```python
from build123d import *

# Parameters (mm, degrees)
BOSS_EXTRUDE2_DEPTH = 21.59
CUT_EXTRUDE1_DEPTH  = 17.78
BOSS_EXTRUDE4_DEPTH = 2.54
SKETCH8_R           = 1.905
CUT_EXTRUDE2_DEPTH  = 2.54
BOSS_EXTRUDE6_DEPTH = 2.54
FILLET1_R           = 2.54
SKETCH13_W          = 19.05
SKETCH13_H          = 2.54
CUT_EXTRUDE5_DEPTH  = 1.27
CUT_EXTRUDE6_DEPTH  = 1.27
SKETCH16_W          = 19.05
SKETCH16_H          = 2.54
CUT_EXTRUDE7_DEPTH  = 1.27
SKETCH17_R          = 8.89
BOSS_EXTRUDE7_DEPTH = 21.844
FILLET2_R           = 2.54


with BuildPart() as part:
    # Sketch3 → Boss-Extrude2 (new body)
    with BuildSketch(Plane.XY):
        with BuildLine():
            Line((-22.77090231, 76.154735329), (22.77090231, 76.154735329))
            ThreePointArc((22.77090231, 76.154735329), (24.597640016, 75.379566583), (25.309393487, 73.527199387))
            Line((25.309393487, 73.527199387), (22.858491178, 2.452464058))
            ThreePointArc((22.858491178, 2.452464058), (22.084831254, 0.713262294), (20.32, 0))
            Line((20.32, 0), (-20.32, 0))
            ThreePointArc((-20.32, 0), (-22.084831254, 0.713262294), (-22.858491178, 2.452464058))
            Line((-22.858491178, 2.452464058), (-25.309393487, 73.527199387))
            ThreePointArc((-25.309393487, 73.527199387), (-24.597640016, 75.379566583), (-22.77090231, 76.154735329))
        make_face()
    extrude(amount=BOSS_EXTRUDE2_DEPTH)

    # Sketch4 → Cut-Extrude1 (cut)
    with BuildSketch(Plane.XY.offset(21.59)):
        with BuildLine():
            Line((-19.541270744, 73.614735329), (20.141804619, 73.614735329))
            ThreePointArc((20.141804619, 73.614735329), (21.968542325, 72.839566583), (22.680295797, 70.987199387))
            Line((22.680295797, 70.987199387), (20.404569365, 4.992462187))
            ThreePointArc((20.404569365, 4.992462187), (19.630909441, 3.253260423), (17.866078187, 2.539998129))
            Line((17.866078187, 2.539998129), (-18.061159176, 2.539998129))
            ThreePointArc((-18.061159176, 2.539998129), (-19.78310781, 3.39559701), (-20.412160003, 5.212586245))
            Line((-20.412160003, 5.212586245), (-22.687990425, 71.210339105))
            ThreePointArc((-22.687990425, 71.210339105), (-21.690891162, 73.166710129), (-19.541270744, 73.614735329))
        make_face()
    extrude(amount=-CUT_EXTRUDE1_DEPTH, mode=Mode.SUBTRACT)

    # Sketch7 → Boss-Extrude4 (add)
    with BuildSketch(Plane.XY.offset(21.59)):
        Polygon((-21.717608556, 43.069831723), (-8.531459132, 43.069831723), (-8.531459132, 32.909831723), (-21.367256671, 32.909831723), align=None)
        Polygon((8.531459132, 32.909831723), (21.367256671, 32.909831723), (21.717608556, 43.069831723), (8.531459132, 43.069831723), align=None)
    extrude(amount=-BOSS_EXTRUDE4_DEPTH)

    # Sketch8 → Cut-Extrude2 (cut)
    with BuildSketch(Plane.XY.offset(21.59)):
        with Locations((-15.036945873, 37.989831723)):
            Circle(SKETCH8_R)
        with Locations((15.237744036, 37.820383377)):
            Circle(SKETCH8_R)
    extrude(amount=-CUT_EXTRUDE2_DEPTH, mode=Mode.SUBTRACT)

    # Sketch10 → Boss-Extrude6 (add)
    with BuildSketch(Plane.XY.offset(10.795)):
        with BuildLine():
            Line((-19.48633529, 73.614735329), (20.196740073, 73.614735329))
            ThreePointArc((20.196740073, 73.614735329), (22.023477783, 72.839566579), (22.73523125, 70.987199377))
            Line((22.73523125, 70.987199377), (20.459504542, 4.992462177))
            ThreePointArc((20.459504542, 4.992462177), (19.685844615, 3.253260419), (17.921013365, 2.539998129))
            Line((17.921013365, 2.539998129), (-18.006223999, 2.539998129))
            ThreePointArc((-18.006223999, 2.539998129), (-19.816312644, 3.37520138), (-20.468700556, 5.258914571))
            Line((-20.468700556, 5.258914571), (-22.744530979, 71.256667431))
            ThreePointArc((-22.744530979, 71.256667431), (-21.694916693, 73.236386905), (-19.48633529, 73.614735329))
        make_face()
    extrude(amount=BOSS_EXTRUDE6_DEPTH)

    # Fillet1
    fillet1_edges = [part.edges().sort_by_distance(p)[0] for p in [
        (24.083942332, 37.989831723, 0),
        (22.084831254, 0.713262294, 0),
        (0, 0, 0),
        (-22.084831254, 0.713262294, 0),
        (-24.083942332, 37.989831723, 0),
        (-24.597640016, 75.379566583, 0),
        (0, 76.154735329, 0),
        (24.597640016, 75.379566583, 0),
    ]]
    fillet(fillet1_edges, radius=FILLET1_R)

    # Sketch13 → Cut-Extrude5 (cut)
    with BuildSketch(Plane(origin=(22.746873247, -0.784390739, 0), x_dir=(0, 0, -1), z_dir=(0.999405975, -0.034462969, 0))):
        with Locations((-12.065, 47.745550873)):
            Rectangle(SKETCH13_W, SKETCH13_H)
    extrude(amount=-CUT_EXTRUDE5_DEPTH, mode=Mode.SUBTRACT)

    # Sketch14 → Cut-Extrude6 (cut)
    with BuildSketch(Plane(origin=(0, 0, 0), x_dir=(-1, 0, 0), z_dir=(0, 0, -1))):
        Polygon((-21.897084419, 48.274526929), (21.853290434, 48.274526929), (21.853290434, 45.734526929), (-21.809496448, 45.734526929), align=None)
    extrude(amount=-CUT_EXTRUDE6_DEPTH, mode=Mode.SUBTRACT)

    # Sketch16 → Cut-Extrude7 (cut)
    with BuildSketch(Plane(origin=(-22.746873247, -0.784390739, 0), x_dir=(0, 0, 1), z_dir=(-0.999405975, -0.034462969, 0))):
        with Locations((12.065, 47.745550873)):
            Rectangle(SKETCH16_W, SKETCH16_H)
    extrude(amount=-CUT_EXTRUDE7_DEPTH, mode=Mode.SUBTRACT)

    # Sketch17 → Boss-Extrude7 (add)
    with BuildSketch(Plane(origin=(0, 0, 0), x_dir=(-1, 0, 0), z_dir=(0, 0, -1))):
        with Locations((-0.010948496, 60.944631129)):
            Circle(SKETCH17_R)
    extrude(amount=BOSS_EXTRUDE7_DEPTH)

    # Fillet2
    fillet2_edges = [part.edges().sort_by_distance(p)[0] for p in [
        (8.900948496, 60.944631129, 0),
    ]]
    fillet(fillet2_edges, radius=FILLET2_R)


solid = part.part
```
Here's how the part is built. I have some questions about the finished solid (model axes, mm). A direction names the side the tool comes from. Give positions to 0.01 mm unless a question says otherwise; leave off trailing zeros. Order: outer loops, then holes, each group sorted by start corner. A loop starts at its lowest first (then second) coordinate and runs counter-clockwise, first axis right, second up. Notation, with made-up numbers: (58.25, -7.75) -> (103.25, -7.75) arc R28 cw to (103.25, 22.25) -> close; hole circle Ø11 at (3, -27.5). An arc over 180 degrees is marked (long way). Use CSV: the item, a comma, the result in double quotes. Start each with the question number.
Item 1: On a 3-axis mill with a long thin cutter (end or side, diameter ignored), from which of +Z, -Z, +X, -X, +Y, -Y can I reach the whole of each face in a straight line? I mean faces 4 (the flat face through (10, 55, 0)), 5 (the cylindrical face through (-23.338, 38.514, 0.724)), 6 (the cylindrical face through (19.65, 3.27, 17.52)), 7 (the cylindrical face through (19.65, 3.27, 7.35)). Say none if no direction works.
Item 2: I'm going to push flat-ended pins straight in: P1, Ø1.4, axis at x = 4, z = 1, coming from the +Y side; P2, Ø3, axis at x = -15, y = 37, coming from the -Z side; P3, Ø1.3, axis at y = 36, z = 19.5, coming from the +X side. Where does each tip first touch, or does it pass through?
Item 3: Suppose I cut it at A-A (x = 12.5). List the corners of the cut face in (y, z) for me (3 decimals).
Item 4: Suppose I cut it at D-D (z = -14). List the corners of the cut face in (x, y) for me, and give its area (3 significant figures).
Item 5: Suppose I cut it at B-B (z = 5). List the corners of the cut face in (x, y) for me.
Item 6: If I drill on probe 1 along Y at (x, z) = (5, 8); probe 2 along Z at (x, y) = (8, 27) (3 decimals); probe 3 along Z at (x, y) = (-5.5, 48) (3 decimals), over which ranges is the centre line in solid material (lowest first)? Write a range as [from, to].
Item 7: Suppose I cut it at C-C (x = -14.5). List the corners of the cut face in (y, z) for me (3 decimals), and give its area (3 significant figures).
Item 8: Thinking about a two-plate mould opening in X: for faces 1 (the cylindrical face through (21.95, 72.86, 17.52)), 2 (the cylindrical face through (23.3, 37.52, 0.72)), 3 (the flat face through (9, 38, 21.59)), which applies, pulls with the +X half, pulls with the -X half, needs draft (parallel to the pull), parting line crosses it, or undercut?
Answer block:
1,face 4,"-Z"
1,face 5,"-Z, -X, -Y"
1,face 6,"+Z"
1,face 7,"none"
2,P1,"stops at y = 76.01"
2,P2,"stops at z = 0"
2,P3,"stops at x = 24.04"
3,outline,"(0, 2.54) arc R2.54 ccw to (2.54, 0) -> (45.735, 0) -> (45.735, 1.27) -> (48.275, 1.27) -> (48.275, 0) -> (73.615, 0) arc R2.54 ccw to (76.155, 2.54) -> (76.155, 21.59) -> (73.615, 21.59) -> (73.615, 13.335) -> (2.54, 13.335) -> (2.54, 21.59) -> (0, 21.59) -> close; (32.91, 19.05) -> (43.07, 19.05) -> (43.07, 21.59) -> (32.91, 21.59) -> close; hole (2.54, 3.81) -> (73.615, 3.81) -> (73.615, 10.795) -> (2.54, 10.795) -> close"
4,outline,"circle Ø17.78 at (0.01, 60.94)"
4,area,"248 mm^2"
5,outline,"(-25.31, 73.53) -> (-24.44, 48.2) -> (-23.17, 48.25) -> (-23.08, 45.71) -> (-24.35, 45.66) -> (-22.86, 2.45) arc R2.54 ccw to (-20.32, 0) -> (20.32, 0) arc R2.54 ccw to (22.86, 2.45) -> (24.35, 45.66) -> (23.08, 45.71) -> (23.17, 48.25) -> (24.44, 48.2) -> (25.31, 73.53) arc R2.54 ccw to (22.77, 76.15) -> (-22.77, 76.15) arc R2.54 ccw to start; hole (-22.69, 71.21) -> (-20.41, 5.21) arc R2.54 ccw to (-18.06, 2.54) -> (17.87, 2.54) arc R2.54 ccw to (20.4, 4.99) -> (22.68, 70.99) arc R2.54 ccw to (20.14, 73.61) -> (-19.54, 73.61) arc R2.54 ccw to start"
6,probe 1,"y = [0, 2.54], [73.61, 76.15]"
6,probe 2,"z = [0, 3.81], [10.795, 13.335]"
6,probe 3,"z = [1.27, 3.81], [10.795, 13.335]"
7,outline,"(0, 2.54) arc R2.54 ccw to (2.54, 0) -> (45.735, 0) -> (45.735, 1.27) -> (48.275, 1.27) -> (48.275, 0) -> (73.615, 0) arc R2.54 ccw to (76.155, 2.54) -> (76.155, 21.59) -> (73.615, 21.59) -> (73.615, 13.335) -> (2.54, 13.335) -> (2.54, 21.59) -> (0, 21.59) -> close; (32.91, 19.05) -> (36.162, 19.05) -> (36.162, 21.59) -> (32.91, 21.59) -> close; (39.818, 19.05) -> (43.07, 19.05) -> (43.07, 21.59) -> (39.818, 21.59) -> close; hole (2.54, 3.81) -> (73.615, 3.81) -> (73.615, 10.795) -> (2.54, 10.795) -> close"
7,area,"572 mm^2"
8,face 1,"undercut"
8,face 2,"pulls with the +X half"
8,face 3,"needs draft"
